The model under review builds one solid part; all positions refer to its coordinate system, in mm. A direction names the side the tool comes from. Give positions to 0.01 mm unless a question says otherwise; leave off trailing zeros. Loops run counter-clockwise (first coordinate to the right, second up) from the corner with the lowest first, then second, coordinate; pieces in that order, holes last. Notation, with made-up numbers: (-32.75, 66) - (-28.75, 66) arc R18 cw to (-28.75, 79) - close; hole circle Ø8 at (-1, -15). An arc over 180 degrees is marked (long way). Answer as a JSON object with one key per item and string values.
from build123d import *

# Parameters (mm, degrees)
F0_R     = 4.318
F1_DEPTH = 3.175
F2_R     = 3.81
F3_DEPTH = 2.032
F4_R     = 0.79375
F5_DEPTH = 5.208


with BuildPart() as f1:
    # F0 (on Front) → F1 (new body)
    with BuildSketch(Plane.XZ):
        Circle(F0_R)
    extrude(amount=-F1_DEPTH)

    # F2 (on face) → F3 (join)
    with BuildSketch(Plane.XZ):
        Circle(F2_R)
    extrude(amount=F3_DEPTH)

    # F4 (on face) → F5 (cut, through all)
    with BuildSketch(Plane.XZ.offset(2.032)):
        Circle(F4_R)
    extrude(amount=-F5_DEPTH, mode=Mode.SUBTRACT)


solid = f1.part
Q1. Consider section C-C, the plane y = 1. State the section outline as (x, z) points.
Results:
{"outline": "circle Ø8.64 at (0, 0); hole circle Ø1.59 at (0, 0)"}
Q2. Consider section B-B, the plane z = 0. State the section outline as (x, y) points (3 decimals), plus the area to 3 significant figures.
Results:
{"outline": "(-4.318, 0) - (-3.81, 0) - (-3.81, -2.032) - (-0.794, -2.032) - (-0.794, 3.175) - (-4.318, 3.175) - close; (0.794, -2.032) - (3.81, -2.032) - (3.81, 0) - (4.318, 0) - (4.318, 3.175) - (0.794, 3.175) - close", "area": "34.6 mm^2"}
Q3. Clearance check with flat-ended pins moving along their axes: pin 1 Ø3 at (x, y) = (2.5, 0) entering from +Z; pin 2 Ø1 at (x, y) = (-2.5, -1) entering from -Z; pin 3 Ø2.5 at (x, z) = (0, 0) entering from +Y (3 decimals). State where each tip first meets the part, or that it passes through.
Results:
{"pin 1": "stops at z = 4.2", "pin 2": "stops at z = -3.24", "pin 3": "stops at y = 3.175"}
Q4. The part is to be moulded in two halves that separate along Z. For faces 1 (the face through (-0.172, 0.535, -0.775)), 2 (the face through (-0.83, -1, -3.72)), 3 (the face through (0, 3.175, -1)), say which applies: +Z half, -Z half, draft (parallel to the pull), parting line (faces both ways), or undercut.
Results:
{"face 1": "undercut", "face 2": "parting line", "face 3": "draft"}
Q5. To check wall thickness, follow probe 1 along Z at (x, y) = (0, 0.55); probe 2 along Z at (x, y) = (0, -0.9); probe 3 along Y at (x, z) = (4.25, -0.5) (3 decimals). State the ranges of each line that lie inside material, in increasing order. Write a range as [from, to].
Results:
{"probe 1": "z = [-4.32, -0.79], [0.79, 4.32]", "probe 2": "z = [-3.81, -0.79], [0.79, 3.81]", "probe 3": "y = [0, 3.175]"}
Q6. For faces 4 (the face through (0, 0, -4)), 5 (the face through (1, -2.032, 0)), list the 3-axis set-ups (+Z, -Z, +X, -X, +Y, -Y) from which the entire face can be reached by the end or side of a thin tool; tool diameter is ignored.
Results:
{"face 4": "-Y", "face 5": "+Z, -Z, +X, -X, -Y"}
Q7. Consider section D-D, the plane z = 3.25. State the section outline as (x, y) points (3 decimals).
Results:
{"outline": "(-2.843, 0) - (-1.988, 0) - (-1.988, -2.032) - (1.988, -2.032) - (1.988, 0) - (2.843, 0) - (2.843, 3.175) - (-2.843, 3.175) - close"}
Q8. Consider section A-A, the plane x = 0. State the section outline as (y, z) points (3 decimals), plus the area to 3 significant figures.
Results:
{"outline": "(-2.032, -3.81) - (0, -3.81) - (0, -4.318) - (3.175, -4.318) - (3.175, -0.794) - (-2.032, -0.794) - close; (-2.032, 0.794) - (3.175, 0.794) - (3.175, 4.318) - (0, 4.318) - (0, 3.81) - (-2.032, 3.81) - close", "area": "34.6 mm^2"}
